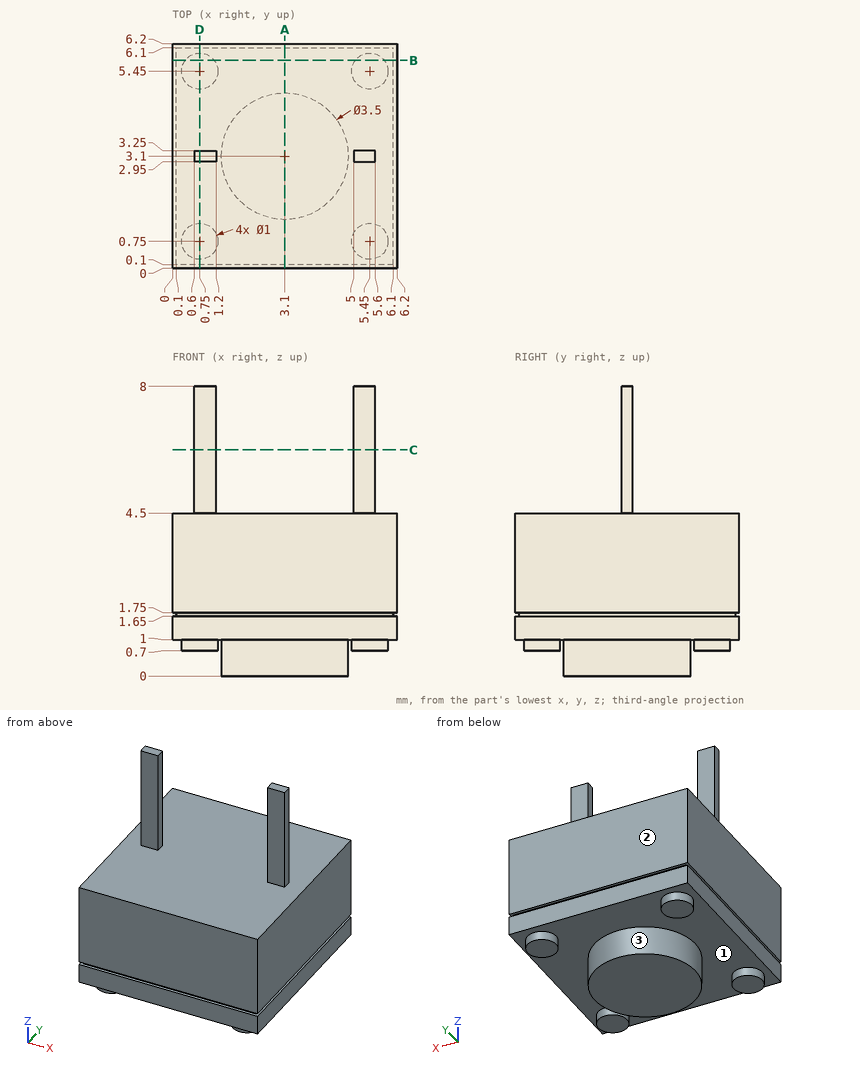
Verification items for this drawing (mm, ordinates from the low corner). Coordinates: 2 decimals unless noted, no trailing zeros. Write each loop counter-clockwise with the first axis right and the second up, starting at its lowest first coordinate (ties: lowest second). Pieces come first, ordered by that corner, then holes. Notation, with made-up numbers: M 6.5,-8.5 L 46.5,-8.5 A19 cw 46.5,27.5 Z; hole C -5,14 d11. An arc over 180 degrees is marked long. Answer as CSV lines item,"result".
Q1. Cross-section at C-C (z = 6.25). Record the boundary of the cut face in (x, y).
Check result:
outline,"M 0.6,2.95 L 1.2,2.95 L 1.2,3.25 L 0.6,3.25 Z; M 5,2.95 L 5.6,2.95 L 5.6,3.25 L 5,3.25 Z"
Q2. Go/stop test with flat-tipped pins: pin 1 (0.5 mm diameter, centred on x = 5, z = 5.5, fed in from -Y); pin 2 (1.1 mm diameter, centred on x = 5.5, y = 5.5, fed in from -Z); pin 3 (0.7 mm diameter, centred on x = 5.5, z = 7, fed in from +Y). Record where each tip stops, or that it passes through.
Check result:
pin 1,"y = 2.95"
pin 2,"z = 0.7"
pin 3,"y = 3.25"
Q3. Cross-section at D-D (x = 0.75). Record the boundary of the cut face in (y, z), then the cut area to 3 significant figures.
Check result:
outline,"M 0,1 L 0.25,1 L 0.25,0.7 L 1.25,0.7 L 1.25,1 L 4.95,1 L 4.95,0.7 L 5.95,0.7 L 5.95,1 L 6.2,1 L 6.2,1.65 L 6.1,1.65 L 6.1,1.75 L 6.2,1.75 L 6.2,4.5 L 3.25,4.5 L 3.25,8 L 2.95,8 L 2.95,4.5 L 0,4.5 L 0,1.75 L 0.1,1.75 L 0.1,1.65 L 0,1.65 Z"
area,"23.3 mm^2"
Q4. Material ranges on probe 1 along Z at (x, y) = (3.5, 3.5); probe 2 along Z at (x, y) = (6, 1.25); probe 3 along Y at (x, z) = (1, 7.25), recorded low to high. Write a range as from..to.
Check result:
probe 1,"0..4.5"
probe 2,"1..4.5"
probe 3,"2.95..3.25"
Q5. Cross-section at B-B (y = 5.75). Record the boundary of the cut face in (x, z).
Check result:
outline,"M 0,1 L 0.35,1 L 0.35,0.7 L 1.15,0.7 L 1.15,1 L 5.05,1 L 5.05,0.7 L 5.85,0.7 L 5.85,1 L 6.2,1 L 6.2,1.65 L 6.1,1.65 L 6.1,1.75 L 6.2,1.75 L 6.2,4.5 L 0,4.5 L 0,1.75 L 0.1,1.75 L 0.1,1.65 L 0,1.65 Z"
Q6. Cross-section at A-A (x = 3.1). Record the boundary of the cut face in (y, z).
Check result:
outline,"M 0,1 L 1.35,1 L 1.35,0 L 4.85,0 L 4.85,1 L 6.2,1 L 6.2,1.65 L 6.1,1.65 L 6.1,1.75 L 6.2,1.75 L 6.2,4.5 L 0,4.5 L 0,1.75 L 0.1,1.75 L 0.1,1.65 L 0,1.65 Z"
Q7. Mould release check, pull along X, two halves, no side actions. Record for the marked faces 1, 2 and 3: released by +X, released by -X, zero draft, split by the parting line, or undercut.
Check result:
face 1,"undercut"
face 2,"zero draft"
face 3,"split by the parting line"
